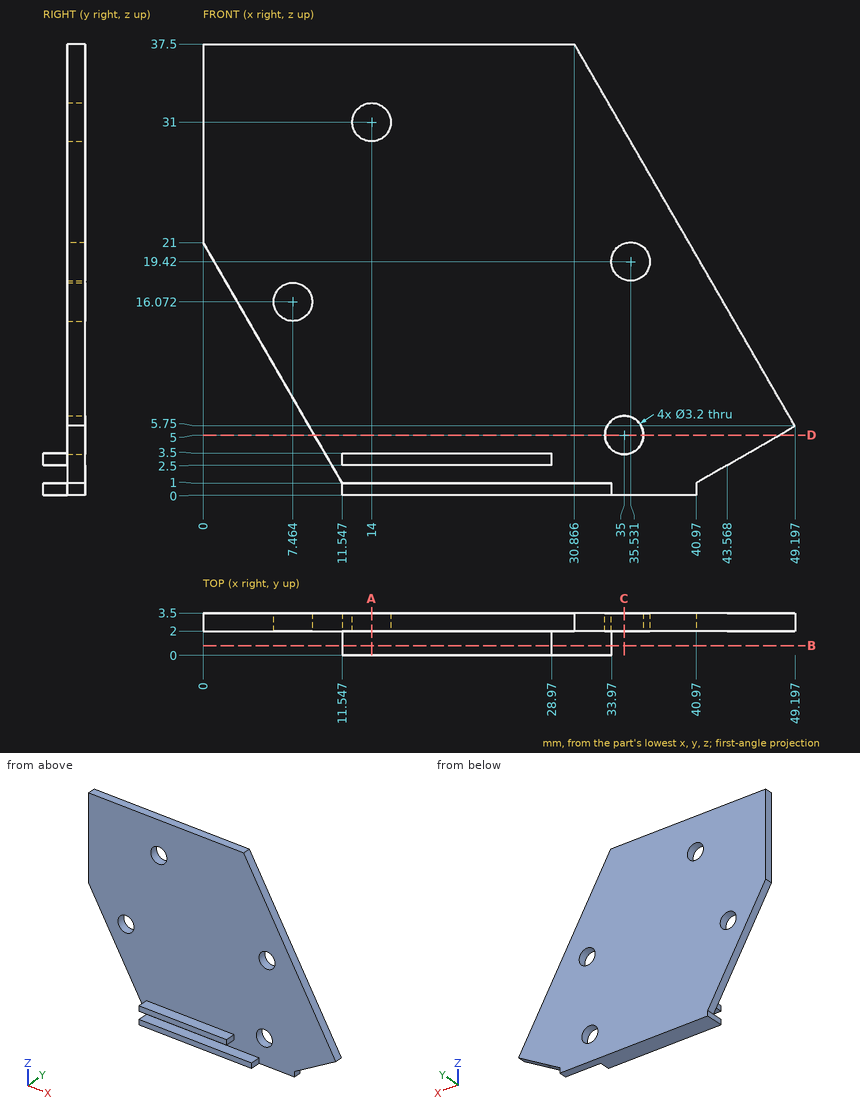
Geometry check sheet. Reference: drawing and pictorial views, mm from the part's lowest x, y, z. Coordinates: 2 decimals unless noted, no trailing zeros. Loops run counter-clockwise (first coordinate to the right, second up) from the corner with the lowest first, then second, coordinate; pieces in that order, holes last. Notation, with made-up numbers: M -25,47 L 32,47 A22 ccw 32,65 Z; hole C 83,19.5 d7. An arc over 180 degrees is marked long. One line per item, written item: value.
1. Section check B-B on y = 0.8. Record the cut outline in (x, z).
Answers follow:
outline: M 11.55,0 L 33.97,0 L 33.97,1 L 11.55,1 Z; M 11.55,2.5 L 28.97,2.5 L 28.97,3.5 L 11.55,3.5 Z
2. Section check C-C on x = 35. Record the cut outline in (y, z).
Answers follow:
outline: M 2,0 L 3.5,0 L 3.5,3.4 L 2,3.4 Z; M 2,6.6 L 3.5,6.6 L 3.5,17.91 L 2,17.91 Z; M 2,20.93 L 3.5,20.93 L 3.5,30.34 L 2,30.34 Z
3. Material ranges on line 1 along Z through (x, y) = (17.5, 0.7); line 2 along Y through (x, z) = (38, 11); line 3 along Z through (x, y) = (29, 1.75), recorded low to high. Write a range as from..to.
Answers follow:
line 1: 0..1, 2.5..3.5
line 2: 2..3.5
line 3: 0..1
4. Section check D-D on z = 5. Record the cut outline in (x, y).
Answers follow:
outline: M 9.24,2 L 33.4,2 L 33.4,3.5 L 9.24,3.5 Z; M 36.6,2 L 47.9,2 L 47.9,3.5 L 36.6,3.5 Z
5. Section check A-A on x = 14. Record the cut outline in (y, z).
Answers follow:
outline: M 0,0 L 3.5,0 L 3.5,29.4 L 2,29.4 L 2,3.5 L 0,3.5 L 0,2.5 L 2,2.5 L 2,1 L 0,1 Z; M 2,32.6 L 3.5,32.6 L 3.5,37.5 L 2,37.5 Z
6. Gauge pin test, flat ends, axial feed: P1, Ø1.5, axis at x = 23, y = 0.5, coming from the +Z side; P2, Ø2, axis at x = 23.5, y = 1.5, coming from the -Z side; P3, Ø1.5, axis at x = 9, y = 1, coming from the +Z side; P4, Ø4, axis at x = 15.5, z = 26, coming from the -Y side. Record the tip position at first contact, or that the pin passes through.
Answers follow:
P1: z = 3.5
P2: z = 0
P3: through
P4: y = 2
